Autodesk Inventor part; units mm, degrees
ref_plane "YZ Plane" through (0, 0, 0) normal (1, 0, 0) x (0, 1, 0)
ref_plane "XZ Plane" through (0, 0, 0) normal (0, 1, 0) x (-1, 0, 0)
ref_plane "XY Plane" through (0, 0, 0) normal (0, 0, 1) x (1, 0, 0)
sketch "Sketch1" plane through (0, 0, 0) normal (0, 0, 1) x (1, 0, 0)
  circle A0 centre (0, 0) radius 2.5
  dimension "Diameter" = 5
extrude "Extrusion1" add sketch "Sketch1" along normal blind 8.9
sketch "Sketch2" plane through (0, 0, 8.9) normal (0, 0, 1) x (1, 0, 0)
  circle A0 centre (0, 0) radius 2.5
extrude "Extrusion2" add sketch "Sketch2" along normal blind 3.1 draft 45
sketch "Sketch3" plane through (0, 0, 12) normal (0, 0, 1) x (1, 0, 0)
  circle A0 centre (0, 0) radius 5.6
  circle A1 centre (0, 0) radius 1.7321 construction
  line L0 (0.725, 1.573) -> (1.7248, 0.1586)
  line L1 (1.7248, 0.1586) -> (0.9997, -1.4144)
  line L2 (0.9997, -1.4144) -> (-0.725, -1.573)
  line L3 (-0.725, -1.573) -> (-1.7248, -0.1586)
  line L4 (-1.7248, -0.1586) -> (-0.9997, 1.4144)
  line L5 (-0.9997, 1.4144) -> (0.725, 1.573)
  dimension "Hex_Width" = 3
extrude "Extrusion3" cut sketch "Sketch3" against normal blind 2 contours L0 L1 L2 L3 L4 L5
thread "Thread1"
chamfer "Chamfer2" distance 0.5 angle 45 1 edges at (-2.5, 0, 0)
fillet "Fillet1" radius 0.1 1 edges at (-5.6, 0, 12)
equation "\"d10\" = Thread_Length"
equation "\"d13\" = Chamfer"
equation "\"Thread_Length\" = 8.9"
equation "\"Length\" = 12"
properties part number "SCREW, FLAT HD, P, 5, M5X0_8X12MM"
The listing builds one solid part. Answer for the finished solid, in the listing's coordinates (mm). A direction names the side the tool comes from. Coordinates: 2 decimals unless noted, no trailing zeros. Loops run counter-clockwise (first coordinate to the right, second up) from the corner with the lowest first, then second, coordinate; pieces in that order, holes last. Notation, with made-up numbers: (70.25, 86) -> (104.25, 86) arc R8 ccw to (104.25, 96) -> close; hole circle Ø7 at (23.5, 68.5). An arc over 180 degrees is marked (long way). Answer in a Markdown table with one row per item. Add a question column.
1. Determine the mould class of faces 1 (the conical face through (2.559, 0.806, 9.083)), 2 (the flat face through (1.367, -0.617, 11.014)), 3 (the flat face through (-1.3, -1.1, 12)) for opening direction X: +X half, -X half, draft (parallel to the pull), parting line (faces both ways), or undercut.
2. The part is cut by section A-A, the plane x = 0. Write down the section's boundary in (y, z).
3. The part is cut by section C-C, the plane y = 0. Write down the section's boundary in (x, z).
4. Consider line 1 (X direction, y = -1.5, z = 1.25); line 2 (Z direction, x = 0.25, y = -1.25); line 3 (Z direction, x = -3, y = 2.25). Determine where each line is inside the solid, lowest interval first. Write a range as [from, to].
5. Flat-ended cylindrical pins translate along their axes: P1, Ø1, axis at x = -1.5, z = 10, coming from the +Y side; P2, Ø1, axis at x = -0.5, y = -1, coming from the -Z side; P3, Ø5, axis at x = 3.5, z = 3.5, coming from the +Y side; P4, Ø6, axis at x = 1, z = 1.5, coming from the -Y side. Find the tip coordinate at first contact, or state that the pin passes through.
6. For faces 4 (the cylindrical face through (-0.54, 2.44, 4.64)), 5 (the flat face through (0, 0, 0)), 6 (the flat face through (0, 0, 10)), determine the directions among +Z, -Z, +X, -X, +Y, -Y from which every point of the face is accessible in a straight line to the end or side of a thin tool.
7. The part is cut by section B-B, the plane z = 2.25. Write down the section's boundary in (x, y), then the cut area to 3 significant figures.
Answer below:
| question | item | result |
|---|---|---|
| 1 | face 1 | parting line |
| 1 | face 2 | undercut |
| 1 | face 3 | draft |
| 2 | outline | (-5.43, 11.83) -> (-2.5, 8.9) -> (-2.5, 0.5) -> (-2, 0) -> (2, 0) -> (2.5, 0.5) -> (2.5, 8.9) -> (5.43, 11.83) arc R0.1 ccw to (5.36, 12) -> (1.51, 12) -> (1.51, 10) -> (-1.51, 10) -> (-1.51, 12) -> (-5.36, 12) arc R0.1 ccw to start |
| 3 | outline | (-5.43, 11.83) -> (-2.5, 8.9) -> (-2.5, 0.5) -> (-2, 0) -> (2, 0) -> (2.5, 0.5) -> (2.5, 8.9) -> (5.43, 11.83) arc R0.1 ccw to (5.36, 12) -> (1.65, 12) -> (1.65, 10) -> (-1.65, 10) -> (-1.65, 12) -> (-5.36, 12) arc R0.1 ccw to start |
| 4 | line 1 | [-2, 2] |
| 4 | line 2 | [0, 10] |
| 4 | line 3 | [10.15, 12] |
| 5 | P1 | y = 3.85 |
| 5 | P2 | z = 0 |
| 5 | P3 | y = 2.29 |
| 5 | P4 | y = -2.5 |
| 6 | face 4 | -Z |
| 6 | face 5 | -Z, +X, -X, +Y, -Y |
| 6 | face 6 | +Z |
| 7 | outline | circle Ø5 at (0, 0) |
| 7 | area | 19.6 mm2 |
